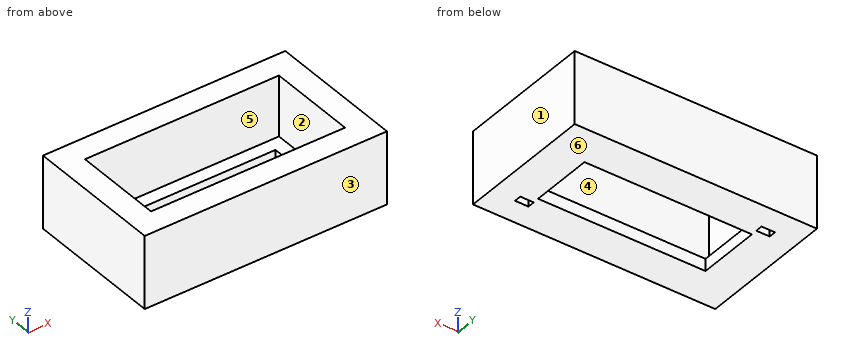
```python
from build123d import *

# Parameters (mm, degrees)
SKETCH1_W           = 20.07
SKETCH1_H           = 11.4
SKETCH1_W_2         = 16.07
SKETCH1_H_2         = 7.4
BOSS_EXTRUDE1_DEPTH = 6
SKETCH2_W           = 16.07
SKETCH2_H           = 7.4
SKETCH2_W_2         = 13.87
SKETCH2_H_2         = 5.2
BOSS_EXTRUDE2_DEPTH = 1
SKETCH3_W           = 1.12
SKETCH3_H           = 0.59
CUT_EXTRUDE1_DEPTH  = 1


with BuildPart() as part:
    # Sketch1 → Boss-Extrude1 (new body)
    with BuildSketch(Plane.XY):
        Rectangle(SKETCH1_W, SKETCH1_H)
        Rectangle(SKETCH1_W_2, SKETCH1_H_2, mode=Mode.SUBTRACT)
    extrude(amount=BOSS_EXTRUDE1_DEPTH)

    # Sketch2 → Boss-Extrude2 (add)
    with BuildSketch(Plane(origin=(0, 0, 0), x_dir=(-1, 0, 0), z_dir=(0, 0, -1))):
        Rectangle(SKETCH2_W, SKETCH2_H)
        Rectangle(SKETCH2_W_2, SKETCH2_H_2, mode=Mode.SUBTRACT)
    extrude(amount=-BOSS_EXTRUDE2_DEPTH)

    # Sketch3 → Cut-Extrude1 (cut)
    with BuildSketch(Plane.XY.offset(1)):
        with Locations((-7.475, 3.405)):
            Rectangle(SKETCH3_W, SKETCH3_H)
        with Locations((7.475, -3.405)):
            Rectangle(SKETCH3_W, SKETCH3_H)
    extrude(amount=-CUT_EXTRUDE1_DEPTH, mode=Mode.SUBTRACT)


solid = part.part
```
The listing builds one solid part. Answer for the finished solid, in the listing's coordinates (mm). Face numbers are marked on the shaded views. A direction names the side the tool comes from. Give positions to 0.01 mm unless a question says otherwise; leave off trailing zeros. Order: outer loops, then holes, each group sorted by start corner. A loop starts at its lowest first (then second) coordinate and runs counter-clockwise, first axis right, second up. Notation, with made-up numbers: (58.5, 82.25) -> (92.5, 82.25) arc R19 cw to (92.5, 95.25) -> close; hole circle Ø5 at (39, 49.25). An arc over 180 degrees is marked (long way). Write each question's results on one line, items separated by ' | '.
Q1. Which of the six approach directions +Z, -Z, +X, -X, +Y, -Y give full straight-line access (tool end or side, diameter ignored) to the marked faces 1 and 2?
Checked values:
face 1: +Z, -Z, +X, +Y, -Y | face 2: +Z
Q2. The part is cut by section C-C, the plane x = 3.25. Give the vertices of the cut face in (y, z).
Checked values:
outline: (-5.7, 0) -> (-2.6, 0) -> (-2.6, 1) -> (-3.7, 1) -> (-3.7, 6) -> (-5.7, 6) -> close; (2.6, 0) -> (5.7, 0) -> (5.7, 6) -> (3.7, 6) -> (3.7, 1) -> (2.6, 1) -> close
Q3. The part is cut by section B-B, the plane y = -1.25. Give the vertices of the cut face in (x, z) (3 decimals), and give its area (3 significant figures).
Checked values:
outline: (-10.035, 0) -> (-6.935, 0) -> (-6.935, 1) -> (-8.035, 1) -> (-8.035, 6) -> (-10.035, 6) -> close; (6.935, 0) -> (10.035, 0) -> (10.035, 6) -> (8.035, 6) -> (8.035, 1) -> (6.935, 1) -> close | area: 26.2 mm^2
Q4. Determine the mould class of the marked faces 3, 4, 5 and 6 for opening direction Y: pulls with the +Y half, pulls with the -Y half, needs draft (parallel to the pull), parting line crosses it, or undercut.
Checked values:
face 3: pulls with the -Y half | face 4: undercut | face 5: undercut | face 6: needs draft
Q5. This flat-tipped pin is pushed along its axis until it touches: P1, Ø3, axis at x = 0.5, y = -2.5, coming from the -Z side. Where does it stop, or does it pass through?
Checked values:
P1: stops at z = 0
Q6. The part is cut by section A-A, the plane z = 2.55. Give the vertices of the cut face in (x, y) (3 decimals).
Checked values:
outline: (-10.035, -5.7) -> (10.035, -5.7) -> (10.035, 5.7) -> (-10.035, 5.7) -> close; hole (-8.035, -3.7) -> (8.035, -3.7) -> (8.035, 3.7) -> (-8.035, 3.7) -> close
Q7. Straight lines are drawn through the part: probe 1 along X at (y, z) = (-1, 3) (3 decimals); probe 2 along Y at (x, z) = (-5, 5.2); probe 3 along X at (y, z) = (-1.5, 0.3) (3 decimals). For each, find the intervals that lie inside material, in ascending order. Write a range as from..to.
Checked values:
probe 1: x = -10.035..-8.035, 8.035..10.035 | probe 2: y = -5.7..-3.7, 3.7..5.7 | probe 3: x = -10.035..-6.935, 6.935..10.035
